Here's the drawing with two shaded views (mm, measured from the low corner). I have some questions. A direction names the side the tool comes from. Round coordinates to 2 decimals unless told otherwise and drop trailing zeros. Order: outer loops, then holes, each group sorted by start corner. A loop starts at its lowest first (then second) coordinate and runs counter-clockwise, first axis right, second up. Notation, with made-up numbers: M 65.5,-10 L 103.5,-10 A24 cw 103.5,22 Z; hole C -2,88 d6. An arc over 180 degrees is marked long. One line per question, with ' | ' between items.
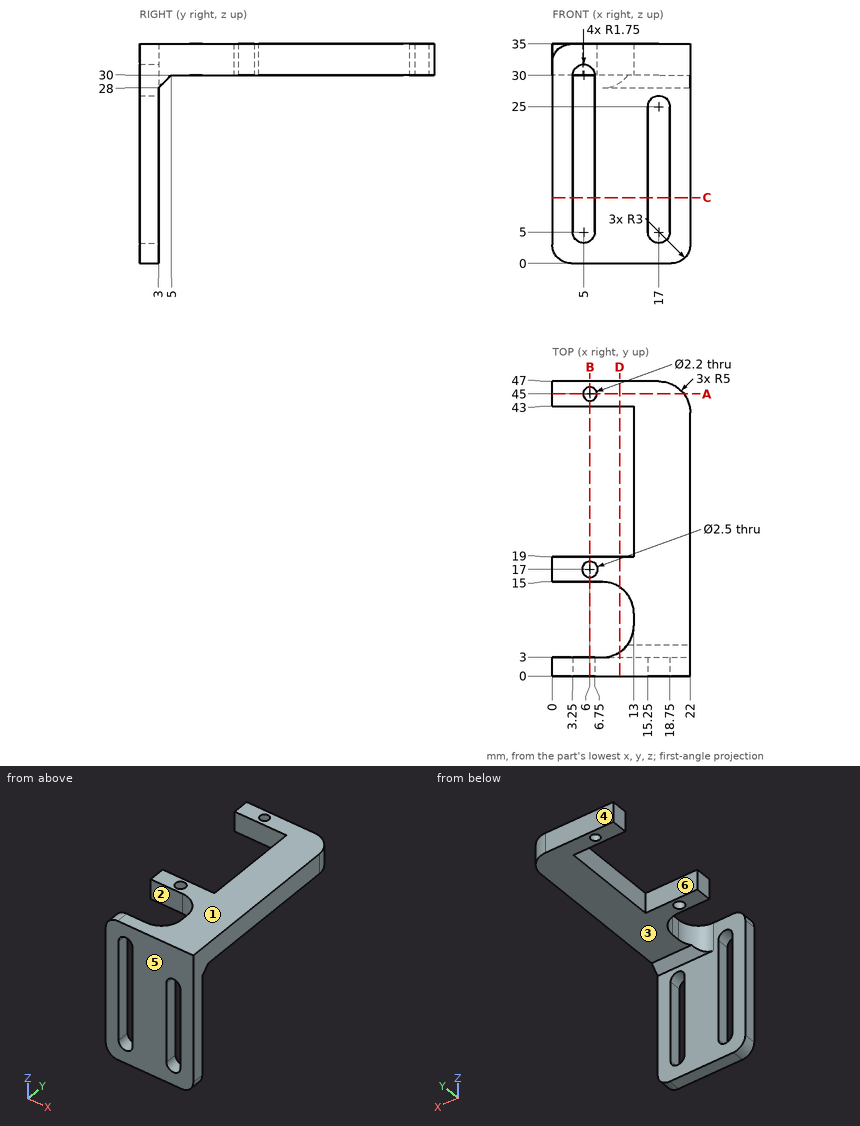
(1) If we section it at A-A on y = 45: Please give me the cut outline in (x, z).
Final values:
outline: M 0,30 L 4.9,30 L 4.9,35 L 0,35 Z; M 7.1,30 L 21,30 L 21,35 L 7.1,35 Z
(2) If we section it at C-C on z = 10.5: Please give me the cut outline in (x, y), plus the area to 3 significant figures.
Final values:
outline: M 0,0 L 3.25,0 L 3.25,3 L 0,3 Z; M 6.75,0 L 15.25,0 L 15.25,3 L 6.75,3 Z; M 18.75,0 L 22,0 L 22,3 L 18.75,3 Z | area: 45.0 mm^2
(3) On a 3-axis mill with a long thin cutter (end or side, diameter ignored), from which of +Z, -Z, +X, -X, +Y, -Y can I reach the whole of each face in a straight line? I mean the marked faces 1, 2 and 3. Say none if no direction works.
Final values:
face 1: +Z, +X, -X, +Y, -Y | face 2: +Z, -Z, -X | face 3: -Z, +X, -X, +Y
(4) If we section it at D-D on x = 10.75: Please give me the cut outline in (y, z).
Final values:
outline: M 0,0 L 3,0 L 3,28 L 3.82,28.82 L 3.82,35 L 0,35 Z; M 14.18,30 L 19,30 L 19,35 L 14.18,35 Z; M 43,30 L 47,30 L 47,35 L 43,35 Z
(5) Thinking about a two-plate mould opening in Y: for the marked faces 4, 5 and 6, which applies, released by +Y, released by -Y, zero draft, split by the parting line, or undercut?
Final values:
face 4: released by +Y | face 5: released by -Y | face 6: undercut
(6) If we section it at B-B on x = 6: Please give me the cut outline in (y, z).
Final values:
outline: M 0,0 L 3,0 L 3,3.56 L 0,3.56 Z; M 0,31.44 L 3,31.44 L 3,35 L 0,35 Z; M 15,30 L 15.75,30 L 15.75,35 L 15,35 Z; M 18.25,30 L 19,30 L 19,35 L 18.25,35 Z; M 43,30 L 43.9,30 L 43.9,35 L 43,35 Z; M 46.1,30 L 47,30 L 47,35 L 46.1,35 Z
(7) Please list where these lines run through material, in increasing order: probe 1 along Y at (x, z) = (6, 33.1); probe 2 along Y at (x, z) = (6, 31.1); probe 3 along X at (y, z) = (2, 5.5). Write a range as [from, to].
Final values:
probe 1: [0, 3], [15, 15.75], [18.25, 19], [43, 43.9], [46.1, 47] | probe 2: [15, 15.75], [18.25, 19], [43, 43.9], [46.1, 47] | probe 3: [0, 3.25], [6.75, 15.25], [18.75, 22]
(8) Will these pins go through, and if not, where does the flat tip stop? pin 1 Ø4 at (y, z) = (31.5, 33) entering from -X; pin 2 Ø3 at (x, y) = (6, 45) entering from -Z; pin 3 Ø10 at (x, z) = (15, 6) entering from +Y.
Final values:
pin 1: x = 13 | pin 2: z = 30 | pin 3: y = 3
